For this review, take the finished solid that the model builds, in its own axes (mm). Face numbers are marked on the shaded views. A direction names the side the tool comes from. Coordinates: 2 decimals unless noted, no trailing zeros. Write each loop counter-clockwise with the first axis right and the second up, starting at its lowest first coordinate (ties: lowest second). Pieces come first, ordered by that corner, then holes. Notation, with made-up numbers: (64.25, -32.75) -> (88.25, -32.75) arc R30 ccw to (88.25, -0.75) -> close; hole circle Ø10 at (82.25, 14.25). An arc over 180 degrees is marked (long way). One line per item, written item: value. Start each with the question number.
1) Mouldability with a two-part tool opening along X and no side actions: class the marked faces 5, 6 and 7 as released by +X, released by -X, zero draft, split by the parting line, or undercut.
2) Add section B-B (x = -4.75). State the section outline as (y, z) points.
3) Add section D-D (x = -1.25). State the section outline as (y, z) points.
4) For probe 1 along X at (y, z) = (-5, 0.6); probe 2 along X at (y, z) = (4.75, 3.4); probe 3 along Y at (x, z) = (4.5, 4.65), list the stretches that pass through material, from the lowest coordinate up. Write a range as from..to.
5) Machinability: for the marked faces 1, 2, 3 and 4, which of the approach directions +Z, -Z, +X, -X, +Y, -Y give a long, thin tool a straight path to every point of the face, cutting with its end or side? Answer none if there is none.
6) Add section C-C (y = 0.75). State the section outline as (x, z) points.
7) Add section A-A (x = -3.5). State the section outline as (y, z) points.
8) For pin 1 Ø1 at (x, z) = (-3.5, 4.5) entering from -Y, flat-tipped, find the tip position at first contact; note if it passes through.
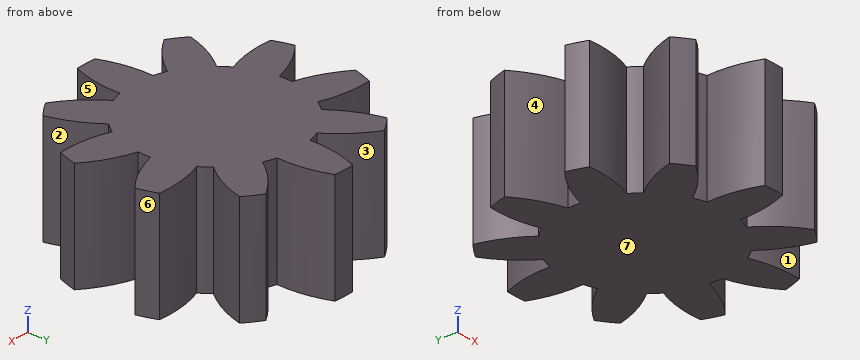
Autodesk Inventor part; units mm, degrees
ref_plane "Work Plane2" through (0, 0, 2.5) normal (0, 0, 1) x (1, 0, 0)
ref_plane "Work Plane8" through (0, 0, 0) normal (0.9510565, 0.309017, 0) x (0, 0, 1)
ref_plane "Work Plane9" through (0, 0, 0) normal (1, 0, 0) x (0, 1, 0)
sketch "Sketch1" plane through (0, 0, 0) normal (0, 0, 1) x (1, 0, 0)
  circle A0 centre (0, 0) radius 6
  dimension "d0" = 12
extrude "Extrusion1" add sketch "Sketch1" along normal blind 5
ref_plane "Work Plane2" through (0, 0, 2.5) normal (0, 0, 1) x (1, 0, 0)
sketch "Sketch2" plane through (0, 0, 0) normal (0, 0, -1) x (-1, 0, 0)
  circle A0 centre (0, 0) radius 6
  circle A1 centre (0, 0) radius 5
  dimension "d3" = 10
surface extrude "Diámetro de separación" sketch "Sketch2" against normal through all shown no curves A1
ref_plane "Work Plane8" through (0, 0, 0) normal (0.9510565, 0.309017, 0) x (0, 0, 1)
ref_plane "Work Plane9" through (0, 0, 0) normal (1, 0, 0) x (0, 1, 0)
spur gear teeth "Engranaje recto" teeth 10 pitch diameter 10 tip diameter 12 root diameter 7.5 face width 5 start plane through (0, 0, 0) normal (0, 0, -1) x (-1, 0, 0)
equation "\"d0\" = da_da"
equation "\"d1\" = da_b"
equation "\"d3\" = da_d"
properties part number "Engranaje recto1" material "Steel"
Numbers:
1. face 5: undercut
1. face 6: released by +X
1. face 7: zero draft
2. outline: (-2.3, 0) -> (-0.68, 0) -> (-0.68, 5) -> (-2.3, 5) -> close; (0.68, 0) -> (2.3, 0) -> (2.3, 5) -> (0.68, 5) -> close
3. outline: (-3.54, 0) -> (3.54, 0) -> (3.54, 5) -> (-3.54, 5) -> close
4. probe 1: -3.32..-2.96, -0.77..0.77, 2.96..3.32
4. probe 2: -3.67..-2.61, -0.82..0.82, 2.61..3.67
4. probe 3: -2.28..-0.56, 0.56..2.28
5. face 1: +Z, -Z
5. face 2: +Z, -Z, +X
5. face 3: +Z, -Z, +Y
5. face 4: +Z, -Z, -X
6. outline: (-4.88, 0) -> (4.88, 0) -> (4.88, 5) -> (-4.88, 5) -> close
7. outline: (-4.87, 0) -> (-3.46, 0) -> (-3.46, 5) -> (-4.87, 5) -> close; (-2.06, 0) -> (2.06, 0) -> (2.06, 5) -> (-2.06, 5) -> close; (3.46, 0) -> (4.87, 0) -> (4.87, 5) -> (3.46, 5) -> close
8. pin 1: y = -5.12
